from build123d import *

# Parameters (mm, degrees)
SKETCH1_R           = 1.875
BOSS_EXTRUDE1_DEPTH = 10
SKETCH3_R           = 0.579460837
CUT_EXTRUDE1_DEPTH  = 1


with BuildPart() as part:
    # Sketch1 → Boss-Extrude1 (new body)
    with BuildSketch(Plane(origin=(82.969208633, 0, 0), x_dir=(0, 0, -1), z_dir=(1, 0, 0))):
        with Locations((-223, 21.8)):
            Circle(SKETCH1_R)
    extrude(amount=-BOSS_EXTRUDE1_DEPTH)

    # Sketch2 → Revolve1 (revolve)
    with BuildSketch(Plane.XY.offset(223), mode=Mode.PRIVATE) as revolve1_sk:
        with BuildLine():
            Line((83.847534734, 21.8), (82.969208633, 21.8))
            Line((82.969208633, 21.8), (82.969208633, 19.925))
            Line((82.969208633, 19.925), (82.969208633, 18.993573117))
            ThreePointArc((82.969208633, 18.993573117), (83.620019841, 20.02358109), (83.847534734, 21.220539163))
            Line((83.847534734, 21.220539163), (83.847534734, 21.8))
        make_face()
    revolve(revolve1_sk.sketch.rotate(Axis((82.969208633, 21.8, 223), (1, 0, 0)), 270), axis=Axis((82.969208633, 21.8, 223), (1, 0, 0)))

    # Sketch3 → Cut-Extrude1 (cut)
    with BuildSketch(Plane(origin=(83.847534734, 0, 0), x_dir=(0, 0, -1), z_dir=(1, 0, 0))):
        with Locations((-223, 21.8)):
            Circle(SKETCH3_R)
    extrude(amount=-CUT_EXTRUDE1_DEPTH, mode=Mode.SUBTRACT)


solid = part.part
Can you work these out from the model? Positions are in its coordinate system, mm. A direction names the side the tool comes from. Coordinates: 2 decimals unless noted, no trailing zeros. Write each loop counter-clockwise with the first axis right and the second up, starting at its lowest first coordinate (ties: lowest second). Pieces come first, ordered by that corner, then holes. Notation, with made-up numbers: (-29, 42) -> (-24, 42) arc R23 cw to (-24, 67) -> close; hole circle Ø11 at (37, 32.25). An arc over 180 degrees is marked (long way). Write each question's results on one line, items separated by ' | '. Start each with the question number.
Item 1: On a 3-axis mill with a long thin cutter (end or side, diameter ignored), from which of +Z, -Z, +X, -X, +Y, -Y can I reach the whole of each face in a straight line? I mean faces 1 (the flat face through (82.969, 24, 222)), 2 (the cylindrical face through (83.35, 21.83, 223.58)). Say none if no direction works.
Item 2: I'm going to push flat-ended pins straight in: P1, Ø1.5, axis at y = 23.5, z = 223, coming from the +X side; P2, Ø2, axis at x = 79.5, z = 221, coming from the -Y side; P3, Ø3, axis at x = 78, z = 221, coming from the -Y side. Where does each tip first touch, or does it pass through?
Item 3: If we section it at A-A, the plane x = 78.75: Write out the boundary of the cut face in (y, z) (3 decimals), and give its area (3 significant figures).
Item 4: Thinking about a two-plate mould opening in Y: for faces 3 (the flat face through (82.848, 22, 223)), 4 (the cylindrical face through (78.04, 22.36, 221.21)), 5 (the flat face through (72.969, 22, 223)), which applies, released by +Y, released by -Y, zero draft, split by the parting line, or undercut?
Item 5: Please list where these lines run through material, in increasing order: probe 1 along Y at (x, z) = (83.3, 223); probe 2 along X at (y, z) = (20.6, 224); probe 3 along Y at (x, z) = (74.25, 224.6).
Answer block:
1) face 1: -X | face 2: +X
2) P1: x = 83.83 | P2: y = 20.21 | P3: y = 19.99
3) outline: circle Ø3.75 at (21.8, 223) | area: 11.0 mm²
4) face 3: undercut | face 4: split by the parting line | face 5: zero draft
5) probe 1: 19.41 to 21.22, 22.38 to 24.19 | probe 2: 72.97 to 83.7 | probe 3: 20.82 to 22.78
